from build123d import *

# Parameters (mm, degrees)
CHAMFER1_SIZE = 2
CHAMFER2_SIZE = 1


with BuildPart() as part:
    # Sketch1 → Revolve1 (revolve)
    with BuildSketch(Plane.XY):
        Polygon((-7.5, -20.5), (-7.5, -30), (-2, -30), (-2, -20.5), (-2.5, -20.5), (-2.5, 17), (-6.5, 17), (-6.5, 0), (-11, 0), (-11, -20.5), align=None)
    revolve(axis=Axis((0, -30, 0), (0, 1, 0)))

    # Chamfer1
    chamfer1_edges = [part.edges().sort_by_distance(p)[0] for p in [
        (7.5, -30, 0),
    ]]
    chamfer(chamfer1_edges, length=CHAMFER1_SIZE)

    # Chamfer2
    chamfer2_edges = [part.edges().sort_by_distance(p)[0] for p in [
        (11, -20.5, 0),
    ]]
    chamfer(chamfer2_edges, length=CHAMFER2_SIZE)


solid = part.part
Here's how the part is built. I have some questions about the finished solid (model axes, mm). A direction names the side the tool comes from. Round coordinates to 2 decimals unless told otherwise and drop trailing zeros. Loops run counter-clockwise (first coordinate to the right, second up) from the corner with the lowest first, then second, coordinate; pieces in that order, holes last. Notation, with made-up numbers: (6.25, -27.75) -> (30.25, -27.75) arc R11 ccw to (30.25, -17.75) -> close; hole circle Ø2 at (79, 54). An arc over 180 degrees is marked (long way). Write each question's results on one line, items separated by ' | '.
(1) We'd pull the mould along X, two halves only. Please class faces 4 (the face through (0.1, -30, -2.4)), 5 (the face through (0.54, -1.49, -2.44)), 6 (the face through (-1, -20.5, 2)), 7 (the face through (7.493, -24.303, 0.33)): released by +X, released by -X, zero draft, split by the parting line, or undercut.
Worked answers:
face 4: zero draft | face 5: undercut | face 6: undercut | face 7: split by the parting line
(2) For P1, Ø3, axis at x = 3, z = 7.5, coming from the +Y side; P2, Ø8, axis at x = -7, y = 0.5, coming from the +Z side; P3, Ø5, axis at x = 0, z = 0, coming from the -Y side; P4, Ø3, axis at x = -3, y = -25, coming from the +Z side, each with a flat end and sliding along its axis, tell me the tip position at first contact or that it passes through.
Worked answers:
P1: y = 0 | P2: z = 10.57 | P3: y = -30 | P4: z = 7.35
(3) For faces 1 (the face through (5, 0, -5)), 2 (the face through (3, 17, 0)), 3 (the face through (-4, -20.5, 7)), which set-ups out of +Z, -Z, +X, -X, +Y, -Y let a thin tool reach every point of the face, with its end or its side?
Worked answers:
face 1: +Y | face 2: +Z, -Z, +X, -X, +Y | face 3: -Y
(4) If we section it at A-A, the plane x = 0: List the corners of the cut face in (y, z) for me.
Worked answers:
outline: (-30, -5.5) -> (-28, -7.5) -> (-20.5, -7.5) -> (-20.5, -10) -> (-19.5, -11) -> (0, -11) -> (0, -6.5) -> (17, -6.5) -> (17, -2.5) -> (-20.5, -2.5) -> (-20.5, -2) -> (-30, -2) -> close; (-30, 2) -> (-20.5, 2) -> (-20.5, 2.5) -> (17, 2.5) -> (17, 6.5) -> (0, 6.5) -> (0, 11) -> (-19.5, 11) -> (-20.5, 10) -> (-20.5, 7.5) -> (-28, 7.5) -> (-30, 5.5) -> close
(5) If we section it at B-B, the plane y = -3.5: List the corners of the cut face in (x, z) for me.
Worked answers:
outline: circle Ø22 at (0, 0); hole circle Ø5 at (0, 0)
(6) If we section it at C-C, the plane y = -27: List the corners of the cut face in (x, z) for me.
Worked answers:
outline: circle Ø15 at (0, 0); hole circle Ø4 at (0, 0)
(7) If I drill on L1, parallel to Z at x = 0, y = -11; L2, parallel to Z at x = 0, y = -26.75; L3, parallel to Y at x = 7.5, z = 0.75, over which ranges is the centre line in solid material (lowest first)?
Worked answers:
L1: -11 to -2.5, 2.5 to 11 | L2: -7.5 to -2, 2 to 7.5 | L3: -20.5 to 0
